Verification items for the finished model (mm, model axes). A direction names the side the tool comes from. Coordinates: 2 decimals unless noted, no trailing zeros. Loops run counter-clockwise (first coordinate to the right, second up) from the corner with the lowest first, then second, coordinate; pieces in that order, holes last.
Q1. Sectioned sample at B-B (y = 15). Enter the section's corners in (x, z), then the cut area to 3 significant figures.
Q2. Sectioned sample at A-A (z = 8.5). Enter the section's corners in (x, y).
Q3. Mould release check, pull along X, two halves, no side actions. Record for faces 1 (the face through (25, 0, 5)), 2 (the face through (-11.5, 5.9, 0)), 3 (the face through (8.766, 8.911, 4.93)), 4 (the face through (15, -2.5, 5)): +X half, -X half, draft (parallel to the pull), parting line (faces both ways), or undercut.
Q4. Material ranges on probe 1 along Y at (x, z) = (12.5, 5.5); probe 2 along Y at (x, z) = (2, 4), recorded low to high.
Q5. Sectioned sample at C-C (x = -5). Enter the section's corners in (y, z), then the cut area to 3 significant figures.
Q6. Access from +Z, -Z, +X, -X, +Y, -Y to the whole of each face (thin tool, end or side, straight path). Record for faces 5 (the face through (15, 2.5, 5)), 6 (the face through (-11.5, 5.9, 10)).
```python
from build123d import *

# Parameters (mm, degrees)
F0_W     = 50
F0_H     = 50
F1_DEPTH = 10


with BuildPart() as f1:
    # F0 (on Top) → F1 (new body)
    with BuildSketch(Plane.XY):
        Rectangle(F0_W, F0_H)
        with BuildLine():
            ThreePointArc((2.5, 17.3205080757), (12.3743686708, 12.3743686708), (17.3205080757, 2.5))
            Line((17.3205080757, 2.5), (21.1176965386, 2.5))
            Line((21.1176965386, 2.5), (21.1176965386, -2.5))
            Line((21.1176965386, -2.5), (17.3205080757, -2.5))
            ThreePointArc((17.3205080757, -2.5), (12.3743686708, -12.3743686708), (2.5, -17.3205080757))
            Line((2.5, -17.3205080757), (2.5, -18.6099875718))
            Line((2.5, -18.6099875718), (-2.5, -18.6099875718))
            Line((-2.5, -18.6099875718), (-2.5, -17.3205080757))
            ThreePointArc((-2.5, -17.3205080757), (-12.3743686708, -12.3743686708), (-17.3205080757, -2.5))
            Line((-17.3205080757, -2.5), (-21.1176965386, -2.5))
            Line((-21.1176965386, -2.5), (-21.1176965386, 2.5))
            Line((-21.1176965386, 2.5), (-17.3205080757, 2.5))
            ThreePointArc((-17.3205080757, 2.5), (-12.3743686708, 12.3743686708), (-2.5, 17.3205080757))
            Line((-2.5, 17.3205080757), (-2.5, 18.6099875718))
            Line((-2.5, 18.6099875718), (2.5, 18.6099875718))
            Line((2.5, 18.6099875718), (2.5, 17.3205080757))
        make_face(mode=Mode.SUBTRACT)
        with BuildLine():
            ThreePointArc((-2.5, 17.3205080757), (0, 17.5), (2.5, 17.3205080757))
            Line((2.5, 17.3205080757), (2.5, 18.6099875718))
            Line((2.5, 18.6099875718), (-2.5, 18.6099875718))
            Line((-2.5, 18.6099875718), (-2.5, 17.3205080757))
        make_face()
        with BuildLine():
            ThreePointArc((-17.3205080757, -2.5), (-17.5, 0), (-17.3205080757, 2.5))
            Line((-17.3205080757, 2.5), (-21.1176965386, 2.5))
            Line((-21.1176965386, 2.5), (-21.1176965386, -2.5))
            Line((-21.1176965386, -2.5), (-17.3205080757, -2.5))
        make_face()
        with BuildLine():
            Line((2.5, -18.6099875718), (2.5, -17.3205080757))
            ThreePointArc((2.5, -17.3205080757), (0, -17.5), (-2.5, -17.3205080757))
            Line((-2.5, -17.3205080757), (-2.5, -18.6099875718))
            Line((-2.5, -18.6099875718), (2.5, -18.6099875718))
        make_face()
        with BuildLine():
            Line((21.1176965386, 2.5), (17.3205080757, 2.5))
            ThreePointArc((17.3205080757, 2.5), (17.4550693399, 1.2532175939), (17.5, 0))
            ThreePointArc((17.5, 0), (17.4550693399, -1.2532175939), (17.3205080757, -2.5))
            Line((17.3205080757, -2.5), (21.1176965386, -2.5))
            Line((21.1176965386, -2.5), (21.1176965386, 2.5))
        make_face()
        with BuildLine():
            ThreePointArc((2.5, 12.2474487139), (8.8388347648, 8.8388347648), (12.2474487139, 2.5))
            Line((12.2474487139, 2.5), (17.3205080757, 2.5))
            ThreePointArc((17.3205080757, 2.5), (12.3743686708, 12.3743686708), (2.5, 17.3205080757))
            Line((2.5, 17.3205080757), (2.5, 12.2474487139))
        make_face()
        with BuildLine():
            Line((17.3205080757, -2.5), (12.2474487139, -2.5))
            ThreePointArc((12.2474487139, -2.5), (8.8388347648, -8.8388347648), (2.5, -12.2474487139))
            Line((2.5, -12.2474487139), (2.5, -17.3205080757))
            ThreePointArc((2.5, -17.3205080757), (12.3743686708, -12.3743686708), (17.3205080757, -2.5))
        make_face()
        with BuildLine():
            Line((2.5, -17.3205080757), (2.5, -12.2474487139))
            ThreePointArc((2.5, -12.2474487139), (0, -12.5), (-2.5, -12.2474487139))
            Line((-2.5, -12.2474487139), (-2.5, -17.3205080757))
            ThreePointArc((-2.5, -17.3205080757), (0, -17.5), (2.5, -17.3205080757))
        make_face()
        with BuildLine():
            Line((-2.5, -17.3205080757), (-2.5, -12.2474487139))
            ThreePointArc((-2.5, -12.2474487139), (-8.8388347648, -8.8388347648), (-12.2474487139, -2.5))
            Line((-12.2474487139, -2.5), (-17.3205080757, -2.5))
            ThreePointArc((-17.3205080757, -2.5), (-12.3743686708, -12.3743686708), (-2.5, -17.3205080757))
        make_face()
        with BuildLine():
            ThreePointArc((-12.2474487139, -2.5), (-12.5, 0), (-12.2474487139, 2.5))
            Line((-12.2474487139, 2.5), (-17.3205080757, 2.5))
            ThreePointArc((-17.3205080757, 2.5), (-17.5, 0), (-17.3205080757, -2.5))
            Line((-17.3205080757, -2.5), (-12.2474487139, -2.5))
        make_face()
        with BuildLine():
            ThreePointArc((-12.2474487139, 2.5), (-8.8388347648, 8.8388347648), (-2.5, 12.2474487139))
            Line((-2.5, 12.2474487139), (-2.5, 17.3205080757))
            ThreePointArc((-2.5, 17.3205080757), (-12.3743686708, 12.3743686708), (-17.3205080757, 2.5))
            Line((-17.3205080757, 2.5), (-12.2474487139, 2.5))
        make_face()
    extrude(amount=F1_DEPTH)


solid = f1.part
```
Geometry check:
1. outline: (-25, 0) - (-2.5, 0) - (-2.5, 10) - (-25, 10) - close; (2.5, 0) - (25, 0) - (25, 10) - (2.5, 10) - close
1. area: 450 mm2
2. outline: (-25, -25) - (25, -25) - (25, 25) - (-25, 25) - close; hole (-2.5, 12.25) arc R12.5 ccw (long way) to (12.25, -2.5) - (17.32, -2.5) arc R17.5 ccw to (17.32, 2.5) - (12.25, 2.5) arc R12.5 ccw to (2.5, 12.25) - (2.5, 17.32) arc R17.5 ccw to (-2.5, 17.32) - close
3. face 1: +X half
3. face 2: draft
3. face 3: undercut
3. face 4: undercut
4. probe 1: y = -25 to -2.5, 2.5 to 25
4. probe 2: y = -25 to -12.34, 17.39 to 25
5. outline: (-25, 0) - (-11.46, 0) - (-11.46, 10) - (-25, 10) - close; (11.46, 0) - (25, 0) - (25, 10) - (11.46, 10) - close
5. area: 271 mm2
6. face 5: +Z, -Z
6. face 6: +Z, +X, -X, +Y, -Y
